Can you work these out from the drawing? Everything is in mm from the part's minimum corner. A direction names the side the tool comes from. Coordinates: 2 decimals unless noted, no trailing zeros. Write each loop counter-clockwise with the first axis right and the second up, starting at its lowest first coordinate (ties: lowest second). Pieces come first, ordered by that corner, then holes. Notation, with made-up numbers: (-37, 47.5) -> (14, 47.5) arc R23 ccw to (14, 78.5) -> close; hole circle Ø10 at (78, 20). An arc over 180 degrees is marked (long way). Use a Markdown table: item, result. Add a question column.
Item 1: If I drill on line 1 along Z through (x, y) = (12, 1.5); line 2 along X through (y, z) = (1, 8.75); line 3 along X through (y, z) = (0.5, 6.75), over which ranges is the centre line in solid material (lowest first)? Write a range as from..to.
Item 2: Imagine slicing it at D-D, the plane z = 1.25. Write out the boundary of the cut face in (x, y), and give its area (3 significant figures).
Item 3: If we mould it in two halves opening along Z, with no side actions, what happens to the marked faces 1, 2 and 3? For each: pulls with the +Z half, pulls with the -Z half, needs draft (parallel to the pull), parting line crosses it, or undercut.
Item 4: Imagine slicing it at C-C, the plane y = 0.8. Write out the boundary of the cut face in (x, z), and give its area (3 significant figures).
Item 5: On a 3-axis mill with a long thin cutter (end or side, diameter ignored), from which of +Z, -Z, +X, -X, +Y, -Y can I reach the whole of each face in a straight line? I mean the marked faces 4 and 5. Say none if no direction works.
Item 6: Imagine slicing it at A-A, the plane x = 9.5. Write out the boundary of the cut face in (y, z), and give its area (3 significant figures).
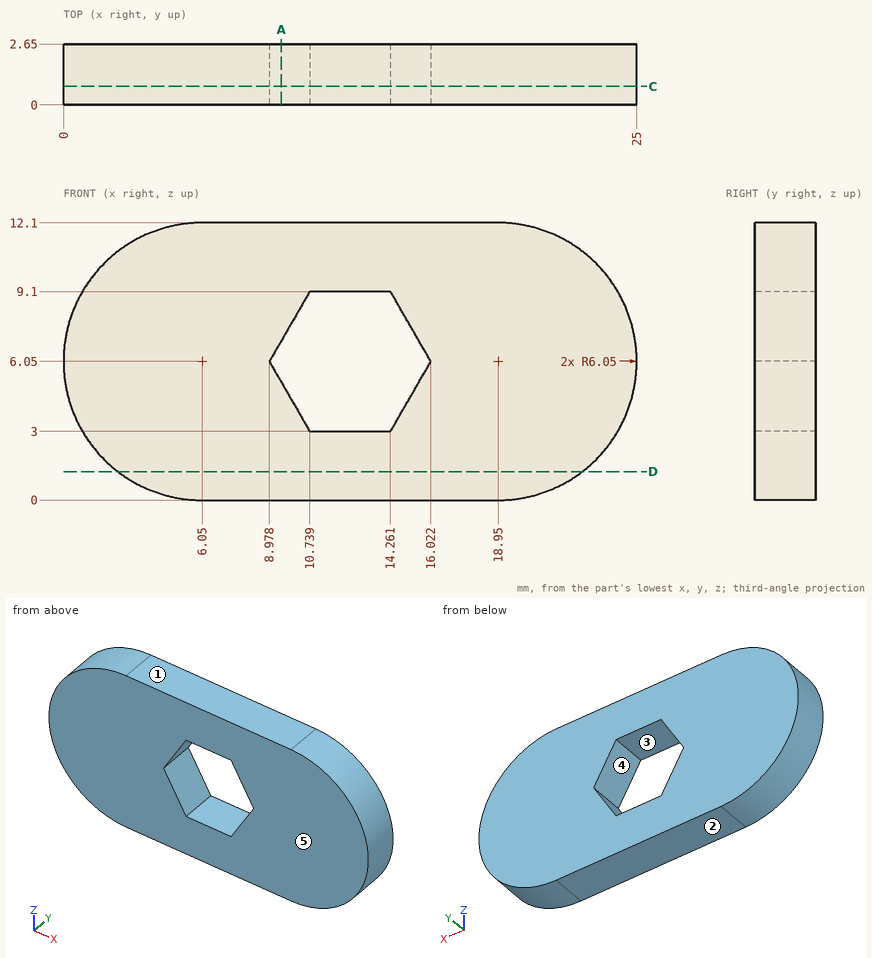
Ans:
| question | item | result |
|---|---|---|
| 1 | line 1 | z = 0..3, 9.1..12.1 |
| 1 | line 2 | x = 0.64..10.54, 14.46..24.36 |
| 1 | line 3 | x = 0.04..9.38, 15.62..24.96 |
| 2 | outline | (2.37, 0) -> (22.63, 0) -> (22.63, 2.65) -> (2.37, 2.65) -> close |
| 2 | area | 53.7 mm^2 |
| 3 | face 1 | pulls with the +Z half |
| 3 | face 2 | pulls with the -Z half |
| 3 | face 3 | undercut |
| 4 | outline | (6.05, 0) -> (18.95, 0) arc R6.05 ccw to (18.95, 12.1) -> (6.05, 12.1) arc R6.05 ccw to start; hole (8.98, 6.05) -> (10.74, 3) -> (14.26, 3) -> (16.02, 6.05) -> (14.26, 9.1) -> (10.74, 9.1) -> close |
| 4 | area | 239 mm^2 |
| 5 | face 4 | +Y, -Y |
| 5 | face 5 | +Z, -Z, +X, -X, -Y |
| 6 | outline | (0, 0) -> (2.65, 0) -> (2.65, 5.15) -> (0, 5.15) -> close; (0, 6.95) -> (2.65, 6.95) -> (2.65, 12.1) -> (0, 12.1) -> close |
| 6 | area | 27.3 mm^2 |
